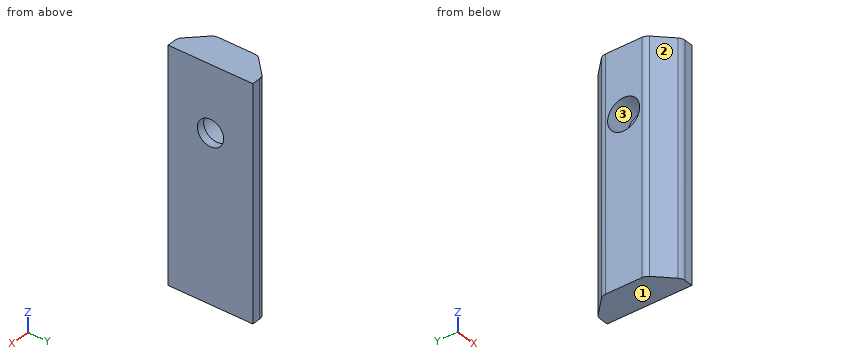
from build123d import *

# Parameters (mm, degrees)
BOSS_EXTRUDE1_DEPTH = 36
SKETCH2_R           = 1.6
CUT_EXTRUDE1_DEPTH  = 10
SKETCH3_R           = 1.95
CUT_EXTRUDE2_DEPTH  = 3
FILLET1_R           = 1
SKETCH4_W           = 8
SKETCH4_H           = 10.3
CUT_EXTRUDE3_DEPTH  = 10


with BuildPart() as part:
    # Sketch1 → Boss-Extrude1 (new body)
    with BuildSketch(Plane.XY):
        Polygon((1.933806537, 5.15), (1.933806537, -5.15), (0.476512405, -5.15), (-2.040358106, -2.633129489), (-2.040358106, 2.633129489), (0.476512405, 5.15), align=None)
    extrude(amount=BOSS_EXTRUDE1_DEPTH)

    # Sketch2 → Cut-Extrude1 (cut)
    with BuildSketch(Plane(origin=(1.933806537, 0, 0), x_dir=(0, 0, -1), z_dir=(1, 0, 0))):
        with Locations((-20, 0)):
            Circle(SKETCH2_R)
        with Locations((-31, 0)):
            Circle(SKETCH2_R)
    extrude(amount=-CUT_EXTRUDE1_DEPTH, mode=Mode.SUBTRACT)

    # Sketch3 → Cut-Extrude2 (cut)
    with BuildSketch(Plane.ZY.offset(2.040358106)):
        with Locations((20, 0)):
            Circle(SKETCH3_R)
        with Locations((31, 0)):
            Circle(SKETCH3_R)
    extrude(amount=-CUT_EXTRUDE2_DEPTH, mode=Mode.SUBTRACT)

    # Fillet1
    fillet1_edges = [part.edges().sort_by_distance(p)[0] for p in [
        (0.476512405, -5.15, 18),
        (-2.040358106, -2.633129489, 18),
        (-2.040358106, 2.633129489, 18),
        (0.476512405, 5.15, 18),
    ]]
    fillet(fillet1_edges, radius=FILLET1_R)

    # Sketch4 → Cut-Extrude3 (cut)
    with BuildSketch(Plane(origin=(1.933806537, 0, 0), x_dir=(0, 0, -1), z_dir=(1, 0, 0))):
        with Locations((-32, 0)):
            Rectangle(SKETCH4_W, SKETCH4_H)
    extrude(amount=-CUT_EXTRUDE3_DEPTH, mode=Mode.SUBTRACT)


solid = part.part
The model under review builds one solid part; all positions refer to its coordinate system, in mm. Face numbers are marked on the shaded views. Coordinates: 2 decimals unless noted, no trailing zeros. Loops run counter-clockwise (first coordinate to the right, second up) from the corner with the lowest first, then second, coordinate; pieces in that order, holes last. Notation, with made-up numbers: M 41.5,-21.75 L 78.5,-21.75 A6 ccw 78.5,-14.75 Z; hole C 20.25,41.5 d7. An arc over 180 degrees is marked long. Put each result on its own line as item: value. Start each with the question number.
Q1. Wall thickness on line 1 (Y direction, x = 1.75, z = 20); line 2 (Y direction, x = 0.1, z = 20); line 3 (Z direction, x = -1.6, y = -0.75): over which ranges is each line inside the solid? List them lowest first.
Q2. Clearance check with a flat-ended pin moving along its axis: pin 1 (3.5 mm diameter, centred on y = 0, z = 20, fed in from -X). State where the tip first meets the part, or that it passes through.
Q3. Add section A-A (y = 0). Write out the cut boundary in (x, z), and give its area (3 significant figures).
Q4. Add section B-B (z = 20). Write out the cut boundary in (x, y), and give its area (3 significant figures).
Q5. The part is to be moulded in two halves that separate along Y. For the marked faces 1, 2 and 3, say which applies: +Y half, -Y half, draft (parallel to the pull), parting line (faces both ways), or undercut.
Q6. Add section C-C (z = 8.75). Write out the cut boundary in (x, y).
Q7. Add section D-D (x = 1.5). Write out the cut boundary in (y, z).
Answers:
1. line 1: y = -5.15 to -1.6, 1.6 to 5.15
1. line 2: y = -4.77 to -1.95, 1.95 to 4.77
1. line 3: z = 0 to 18.2, 21.8 to 28
2. pin 1: stops at x = 0.96
3. outline: M -2.04,0 L 1.93,0 L 1.93,18.4 L 0.96,18.4 L 0.96,18.05 L -2.04,18.05 Z; M -2.04,21.95 L 0.96,21.95 L 0.96,21.6 L 1.93,21.6 L 1.93,28 L -2.04,28 Z
3. area: 96.5 mm^2
4. outline: M -2.04,-2.22 A1 ccw -1.75,-2.93 L 0.18,-4.86 A1 ccw 0.89,-5.15 L 1.93,-5.15 L 1.93,-1.6 L 0.96,-1.6 L 0.96,-1.95 L -2.04,-1.95 Z; M -2.04,1.95 L 0.96,1.95 L 0.96,1.6 L 1.93,1.6 L 1.93,5.15 L 0.89,5.15 A1 ccw 0.18,4.86 L -1.75,2.93 A1 ccw -2.04,2.22 Z
4. area: 19.7 mm^2
5. face 1: draft
5. face 2: -Y half
5. face 3: undercut
6. outline: M -2.04,-2.22 A1 ccw -1.75,-2.93 L 0.18,-4.86 A1 ccw 0.89,-5.15 L 1.93,-5.15 L 1.93,5.15 L 0.89,5.15 A1 ccw 0.18,4.86 L -1.75,2.93 A1 ccw -2.04,2.22 Z
7. outline: M -5.15,0 L 5.15,0 L 5.15,28 L -5.15,28 Z; hole C 0,20 d3.2
